For this review, use the dimensioned drawing (mm, ordinates from the lowest corner) and the shaded views. Round coordinates to 2 decimals unless told otherwise and drop trailing zeros. Order: outer loops, then holes, each group sorted by start corner. A loop starts at its lowest first (then second) coordinate and runs counter-clockwise, first axis right, second up. Notation, with made-up numbers: (14.5, -30.75) -> (68.5, -30.75) arc R28 ccw to (68.5, -6.75) -> close; hole circle Ø2 at (8, 53.25). An arc over 180 degrees is marked (long way). Answer in a Markdown table with one row per item.
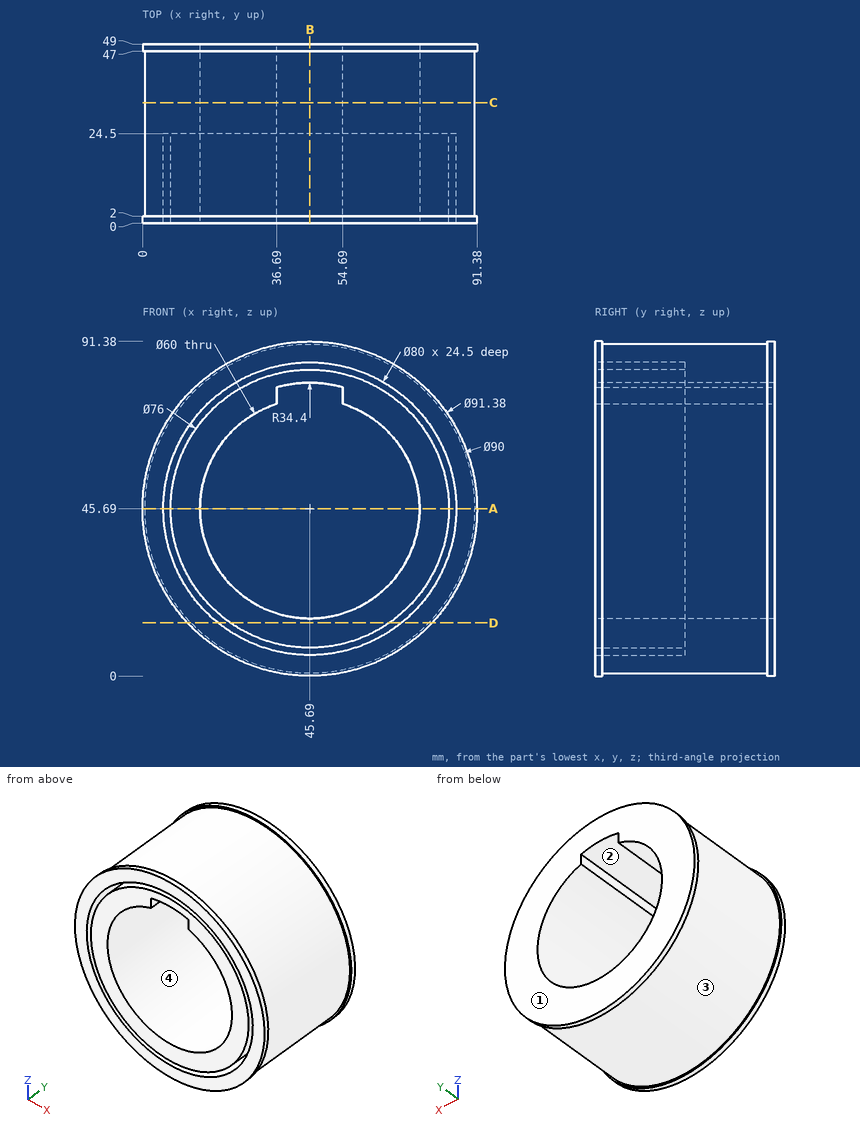
Q1. The part is to be moulded in two halves that separate along X. For the marked faces 1, 2, 3 and 4, say which applies: +X half, -X half, draft (parallel to the pull), parting line (faces both ways), or undercut.
Answer key:
| item | result |
|---|---|
| face 1 | draft |
| face 2 | undercut |
| face 3 | parting line |
| face 4 | undercut |
Q2. Take a section at C-C, the plane y = 33. Write out the cut boundary in (x, z).
Answer key:
| item | result |
|---|---|
| outline | circle Ø90 at (45.69, 45.69); hole (36.69, 74.31) arc R30 ccw (long way) to (54.69, 74.31) -> (54.69, 78.89) arc R34.4 ccw to (36.69, 78.89) -> close |
Q3. Clearance check with flat-ended pins moving along their axes: pin 1 Ø3 at (x, y) = (47, 15) entering from -Z; pin 2 Ø3.5 at (y, z) = (12.5, 75.5) entering from +X; pin 3 Ø1.5 at (y, z) = (16.5, 56) entering from -X. State where each tip first meets the part, or that it passes through.
Answer key:
| item | result |
|---|---|
| pin 1 | stops at z = 0.69 |
| pin 2 | stops at x = 80.87 |
| pin 3 | stops at x = 1.72 |
Q4. To check wall thickness, follow probe 1 along X at (y, z) = (14, 45); probe 2 along Z at (x, y) = (45, 16); probe 3 along Z at (x, y) = (55.5, 12). State the ranges of each line that lie inside material, in increasing order.
Answer key:
| item | result |
|---|---|
| probe 1 | x = 0.7 to 5.7, 7.7 to 15.7, 75.68 to 83.68, 85.68 to 90.68 |
| probe 2 | z = 0.7 to 5.7, 7.7 to 15.7, 80.08 to 83.68, 85.68 to 90.68 |
| probe 3 | z = 1.77 to 6.91, 8.98 to 17.34, 74.04 to 82.4, 84.47 to 89.61 |
Q5. Take a section at B-B, the plane x = 45.69. Write out the cut boundary in (y, z), then the cut area to 3 significant figures.
Answer key:
| item | result |
|---|---|
| outline | (0, 0) -> (2, 0) -> (2, 0.69) -> (47, 0.69) -> (47, 0) -> (49, 0) -> (49, 15.69) -> (0, 15.69) -> (0, 7.69) -> (24.5, 7.69) -> (24.5, 5.69) -> (0, 5.69) -> close; (0, 80.09) -> (49, 80.09) -> (49, 91.38) -> (47, 91.38) -> (47, 90.69) -> (2, 90.69) -> (2, 91.38) -> (0, 91.38) -> (0, 85.69) -> (24.5, 85.69) -> (24.5, 83.69) -> (0, 83.69) -> close |
| area | 1,160 mm^2 |
Q6. Take a section at A-A, the plane z = 45.69. Write out the cut boundary in (x, y).
Answer key:
| item | result |
|---|---|
| outline | (0, 0) -> (5.69, 0) -> (5.69, 24.5) -> (7.69, 24.5) -> (7.69, 0) -> (15.69, 0) -> (15.69, 49) -> (0, 49) -> (0, 47) -> (0.69, 47) -> (0.69, 2) -> (0, 2) -> close; (75.69, 0) -> (83.69, 0) -> (83.69, 24.5) -> (85.69, 24.5) -> (85.69, 0) -> (91.38, 0) -> (91.38, 2) -> (90.69, 2) -> (90.69, 47) -> (91.38, 47) -> (91.38, 49) -> (75.69, 49) -> close |
Q7. Take a section at D-D, the plane z = 14.5. Write out the cut boundary in (x, y), then the cut area to 3 significant figures.
Answer key:
| item | result |
|---|---|
| outline | (12.3, 0) -> (20.65, 0) -> (20.65, 24.5) -> (23.98, 24.5) -> (23.98, 0) -> (67.4, 0) -> (67.4, 24.5) -> (70.73, 24.5) -> (70.73, 0) -> (79.08, 0) -> (79.08, 2) -> (78.13, 2) -> (78.13, 47) -> (79.08, 47) -> (79.08, 49) -> (12.3, 49) -> (12.3, 47) -> (13.25, 47) -> (13.25, 2) -> (12.3, 2) -> close |
| area | 3,020 mm^2 |
